Can you work these out from the drawing? Everything is in mm from the part's minimum corner. A direction names the side the tool comes from. Round coordinates to 2 decimals unless told otherwise and drop trailing zeros. Write each loop counter-clockwise with the first axis right and the second up, starting at its lowest first coordinate (ties: lowest second). Pieces come first, ordered by that corner, then holes. Notation, with made-up numbers: M -18,7.5 L 12,7.5 A20 ccw 12,17.5 Z; hole C 4.5,76 d2. An arc over 180 degrees is marked long. Answer in a Markdown table with one row per item. Add a question column.
(1) If I drill on probe 1 along X at (y, z) = (106, 116); probe 2 along X at (y, z) = (4.5, 11.5); probe 3 along Y at (x, z) = (169, 105), over which ranges is the centre line in solid material (lowest first)?
(2) I'm going to push flat-ended pins straight in: pin 1 (12 mm diameter, centred on x = 20.5, y = 59, fed in from +Z); pin 2 (8 mm diameter, centred on x = 78, z = 58, fed in from +Y); pin 3 (11.5 mm diameter, centred on x = 94.5, z = 8.5, fed in from +Y); pin 4 (7.5 mm diameter, centred on y = 17, z = 35.5, fed in from -X). Where does each tip first touch, or does it pass through?
(3) Suppose I cut it at B-B, the plane z = 11.5. Write out the boundary of the cut face in (x, y).
(4) For the marked faces 1, 2, 3, 4 and 5, which set-ups out of +Z, -Z, +X, -X, +Y, -Y let a thin tool reach every point of the face, with its end or its side?
(5) Suppose I cut it at C-C, the plane y = 99. Write out the boundary of the cut face in (x, z).
(6) Suppose I cut it at D-D, the plane z = 105. Write out the boundary of the cut face in (x, y), then the cut area to 3 significant figures.
(7) If we mould it in two halves opening along X, with no side actions, what happens to the marked faces 6, 7, 8 and 9? For each: released by +X, released by -X, zero draft, split by the parting line, or undercut.
(8) Suppose I cut it at A-A, the plane x = 88. Write out the boundary of the cut face in (y, z).
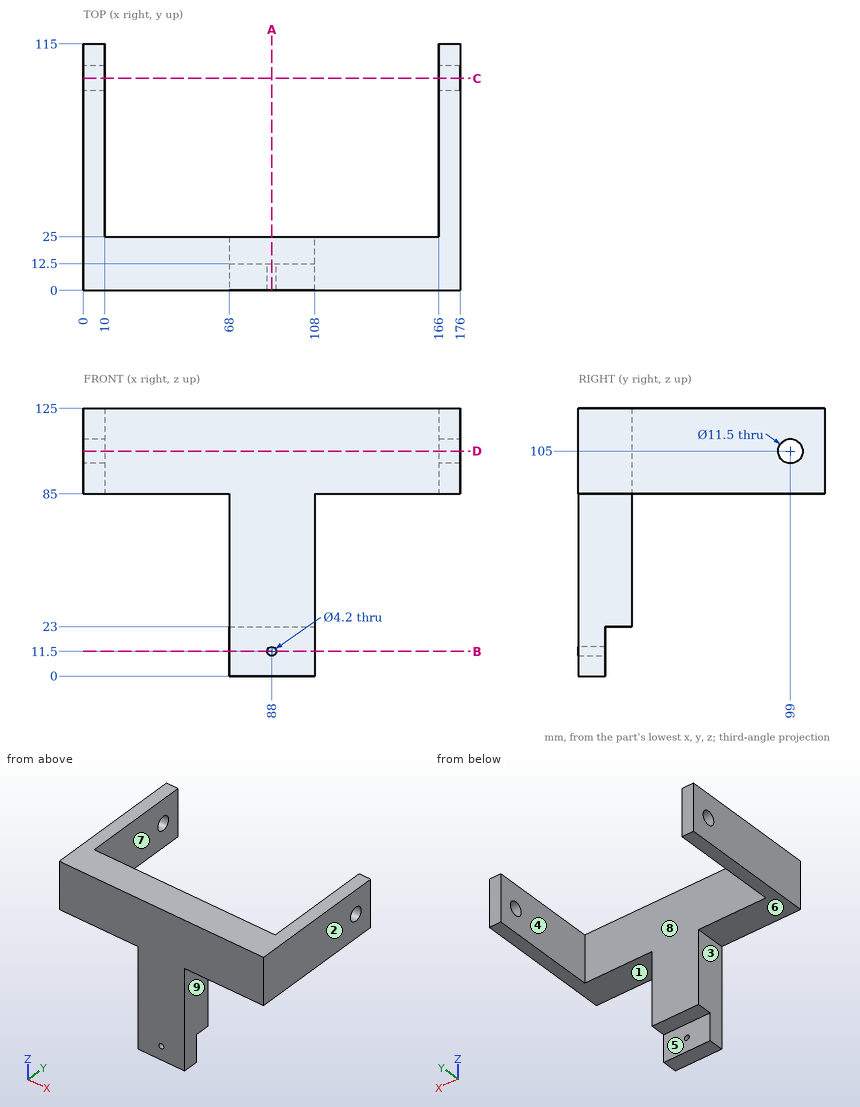
Calculated:
| question | item | result |
|---|---|---|
| 1 | probe 1 | 0 to 10, 166 to 176 |
| 1 | probe 2 | 68 to 85.9, 90.1 to 108 |
| 1 | probe 3 | 0 to 93.25, 104.75 to 115 |
| 2 | pin 1 | through |
| 2 | pin 2 | y = 25 |
| 2 | pin 3 | y = 12.5 |
| 2 | pin 4 | x = 68 |
| 3 | outline | M 68,0 L 85.9,0 L 85.9,12.5 L 68,12.5 Z; M 90.1,0 L 108,0 L 108,12.5 L 90.1,12.5 Z |
| 4 | face 1 | -Z, +X, +Y, -Y |
| 4 | face 2 | +Z, -Z, +X, +Y, -Y |
| 4 | face 3 | -Z, -X, +Y, -Y |
| 4 | face 4 | +Z, -Z, +Y |
| 4 | face 5 | -Z, +X, -X, +Y |
| 5 | outline | M 0,85 L 10,85 L 10,99.25 L 0,99.25 Z; M 0,110.75 L 10,110.75 L 10,125 L 0,125 Z; M 166,85 L 176,85 L 176,99.25 L 166,99.25 Z; M 166,110.75 L 176,110.75 L 176,125 L 166,125 Z |
| 6 | outline | M 0,0 L 176,0 L 176,93.25 L 166,93.25 L 166,25 L 10,25 L 10,93.25 L 0,93.25 Z; M 0,104.75 L 10,104.75 L 10,115 L 0,115 Z; M 166,104.75 L 176,104.75 L 176,115 L 166,115 Z |
| 6 | area | 5,970 mm² |
| 7 | face 6 | zero draft |
| 7 | face 7 | undercut |
| 7 | face 8 | undercut |
| 7 | face 9 | released by +X |
| 8 | outline | M 0,0 L 12.5,0 L 12.5,9.4 L 0,9.4 Z; M 0,13.6 L 12.5,13.6 L 12.5,23 L 25,23 L 25,125 L 0,125 Z |
